The model under review builds one solid part; all positions refer to its coordinate system, in mm. A direction names the side the tool comes from. Give positions to 0.01 mm unless a question says otherwise; leave off trailing zeros. Loops run counter-clockwise (first coordinate to the right, second up) from the corner with the lowest first, then second, coordinate; pieces in that order, holes last. Notation, with made-up numbers: (59.25, 28) -> (66.25, 28) arc R18 cw to (66.25, 50) -> close; hole circle Ø1 at (-28, 72.5). An arc over 180 degrees is marked (long way). Write each question's results on one line, items separated by ' | '. Start each with the question number.
Q1. We need section B-B (y = 7.5). Give the number of separate pieces and of enclosed holes in the cut face, plus the area to 3 significant figures.
Q2. Mouldability with a two-part tool opening along Z and no side actions: class faces 5 (the face through (11, 0, -23)), 6 (the face through (14, 11, 0)), 7 (the face through (13.445, 11.139, -24.225)) as released by +Z, released by -Z, zero draft, split by the parting line, or undercut.
Q3. We need section D-D (x = 11). Write out the cut boundary in (y, z).
Q4. Wall thickness on L1, parallel to Z at x = 18, y = 12.75; L2, parallel to X at y = 22.5, z = -18.5 (3 decimals); L3, parallel to Z at x = 17.5, y = 10: over which ranges is each line inside the solid? List them lowest first. Write a range as [from, to].
Q5. Insertion check: pin 1 Ø5 at (x, z) = (15.5, -35) entering from +Y; pin 2 Ø1.5 at (x, y) = (23.5, 4.5) entering from -Z; pin 3 Ø6 at (x, z) = (20, -42) entering from -Y. Each pin has a flat end and moves straight along its axis. Give the tip position at first contact, or say it passes through.
Q6. Machinability: for faces 1 (the face through (11, 21.971, -23)), 2 (the face through (14, 11, -47.371)), 3 (the face through (28.575, -0.2, -21.7)), 4 (the face through (31.75, 11, -23)), which of the approach directions +Z, -Z, +X, -X, +Y, -Y give a long, thin tool a straight path to every point of the face, cutting with its end or side? Answer none if there is none.
from build123d import *

# Parameters (mm, degrees)
SKETCH1_W           = 47.371
SKETCH1_H           = 21.971
BOSS_EXTRUDE1_DEPTH = 28.575
SKETCH2_W           = 50.8
SKETCH2_H           = 25.4
BOSS_EXTRUDE2_DEPTH = 3.175
CHAMFER1_SIZE       = 0.762
SKETCH3_R           = 2.4892
CUT_EXTRUDE1_DEPTH  = 64.074969049


with BuildPart() as part:
    # Sketch1 → Boss-Extrude1 (new body)
    with BuildSketch(Plane(origin=(0, 0, 0), x_dir=(0, 0, -1), z_dir=(1, 0, 0))):
        with Locations((23.6855, 10.9855)):
            Rectangle(SKETCH1_W, SKETCH1_H)
    extrude(amount=BOSS_EXTRUDE1_DEPTH)

    # Sketch2 → Boss-Extrude2 (add)
    with BuildSketch(Plane(origin=(28.575, 0, 0), x_dir=(0, 0, -1), z_dir=(1, 0, 0))):
        with Locations((23.6855, 10.9855)):
            Rectangle(SKETCH2_W, SKETCH2_H)
    extrude(amount=BOSS_EXTRUDE2_DEPTH)

    # Chamfer1
    chamfer1_edges = [part.edges().sort_by_distance(p)[0] for p in [
        (30.1625, 23.6855, 1.7145),
        (30.1625, -1.7145, 1.7145),
        (30.1625, -1.7145, -49.0855),
        (30.1625, 23.6855, -49.0855),
        (31.75, 10.9855, 1.7145),
        (31.75, -1.7145, -23.6855),
        (31.75, 10.9855, -49.0855),
        (31.75, 23.6855, -23.6855),
        (0, 21.971, -23.6855),
        (0, 10.9855, -47.371),
        (0, 0, -23.6855),
        (0, 10.9855, 0),
        (14.2875, 21.971, 0),
        (14.2875, 21.971, -47.371),
        (14.2875, 0, -47.371),
        (14.2875, 0, 0),
    ]]
    chamfer(chamfer1_edges, length=CHAMFER1_SIZE)

    # Sketch3 → Cut-Extrude1 (cut, through all)
    with BuildSketch(Plane(origin=(0, 21.971, 0), x_dir=(1, 0, 0), z_dir=(0, 1, 0))):
        with Locations(Location((15.875, 23.6855, 0), (0, 0, 270))):
            Circle(SKETCH3_R)
        with Locations(Location((15.875, 36.322, 0), (0, 0, 270))):
            Circle(SKETCH3_R)
        with Locations(Location((15.875, 10.922, 0), (0, 0, 270))):
            Circle(SKETCH3_R)
    extrude(amount=-CUT_EXTRUDE1_DEPTH, mode=Mode.SUBTRACT)


solid = part.part
Output:
1) separate pieces: 1 | enclosed holes: 3 | area: 1,460 mm2
2) face 5: zero draft | face 6: released by +Z | face 7: undercut
3) outline: (0, -46.61) -> (0.76, -47.37) -> (21.21, -47.37) -> (21.97, -46.61) -> (21.97, -0.76) -> (21.21, 0) -> (0.76, 0) -> (0, -0.76) -> close
4) L1: [-47.37, -37.62], [-35.03, -24.98], [-22.39, -12.22], [-9.63, 0] | L2: [28.575, 31.75] | L3: [-47.37, -38.21], [-34.44, -25.57], [-21.8, -12.81], [-9.04, 0]
5) pin 1: y = 21.97 | pin 2: z = -47.37 | pin 3: y = 0
6) face 1: +Z, -Z, -X, +Y | face 2: -Z, -X, +Y, -Y | face 3: -X | face 4: +Z, -Z, +X, +Y, -Y
